Verification items for the finished model (mm, model axes). Face numbers are marked on the shaded views. Round coordinates to 2 decimals unless told otherwise and drop trailing zeros. Order: outer loops, then holes, each group sorted by start corner. A loop starts at its lowest first (then second) coordinate and runs counter-clockwise, first axis right, second up.
Autodesk Inventor part; units mm, degrees
ref_plane "Work Plane6" through (1000, 0, 0) normal (1, 0, 0) x (0, 0, -1)
ref_plane "Work Plane7" through (0, 775, 0) normal (0, 1, 0) x (1, 0, 0)
ref_plane "Work Plane8" through (0, 237, 0) normal (0, -1, 0) x (1, 0, 0)
sketch "Sketch1" plane through (0, 0, 0) normal (0, 0, 1) x (1, 0, 0)
  line L0 (0, 0) -> (1000, 0)
  line L1 (1000, 0) -> (1000, 1000)
  line L2 (1000, 1000) -> (0, 1000)
  line L3 (0, 1000) -> (0, 0)
  dimension "d0" = 1000
  dimension "d1" = 1000
extrude "Extrusion1" add sketch "Sketch1" along normal blind 100
sketch "Sketch8" plane through (0, 0, 100) normal (0, 0, 1) x (1, 0, 0)
  line L0 (1000, 1000) -> (0, 1000)
  line L1 (0, 1000) -> (150, 1000)
  line L2 (150, 1000) -> (150, 850)
  circle A0 centre (150, 850) radius 12.5
  point P0 (0, 0)
  dimension "d30" = 150
  dimension "d31" = 150
  dimension "d32" = 25
extrude "Extrusion4" cut sketch "Sketch8" against normal blind 100
sketch "Sketch9" plane through (0, 0, 100) normal (0, 0, 1) x (1, 0, 0)
  line L0 (425, 260) -> (765, 260)
  line L1 (765, 260) -> (765, 50)
  line L2 (765, 50) -> (425, 50)
  line L3 (425, 50) -> (425, 260)
  line L4 (0, 0) -> (1000, 0)
  line L5 (0, 1000) -> (0, 0)
  dimension "d35" = 210
  dimension "d36" = 340
  dimension "d37" = 50
extrude "Extrusion5" add sketch "Sketch9" along normal blind 115
ref_plane "Work Plane6" through (1000, 0, 0) normal (1, 0, 0) x (0, 0, -1)
ref_plane "Work Plane7" through (0, 775, 0) normal (0, 1, 0) x (1, 0, 0)
sketch "Sketch12" plane through (0, 0, 100) normal (0, 0, 1) x (1, 0, 0)
  line L0 (0, 0) -> (1000, 0)
  line L1 (877, 141) -> (742, 141) construction
  line L2 (877, 141) -> (877, 166) construction
  line L3 (902, 166) -> (902, 116)
  line L4 (902, 116) -> (852, 116)
  line L5 (852, 116) -> (852, 166)
  line L6 (852, 166) -> (902, 166)
  dimension "d58" = 25
  dimension "d59" = 50
  dimension "d60" = 50
  dimension "d63" = 25
  dimension "d64" = 25
extrude "Extrusion8" add sketch "Sketch12" along normal blind 0.5
ref_plane "Work Plane8" through (0, 237, 0) normal (0, -1, 0) x (1, 0, 0)
sketch "Sketch13" plane through (0, 0, 100) normal (0, 0, 1) x (1, 0, 0)
  line L0 (425, 260) -> (425, 50)
  line L1 (425, 155) -> (395, 155)
  line L2 (395, 155) -> (395, 160)
  line L3 (395, 160) -> (220, 160)
  line L4 (220, 160) -> (220, 130)
  line L5 (220, 130) -> (395, 130)
  line L6 (395, 130) -> (395, 155)
  line L7 (425, 50) -> (164, 50)
  point P0 (0, 0)
  dimension "d67" = 30
  dimension "d68" = 5
  dimension "d69" = 175
  dimension "d73" = 80
extrude "Extrusion9" cut sketch "Sketch13" against normal blind 1
sketch "Sketch14" plane through (0, 0, 100) normal (0, 0, 1) x (1, 0, 0)
  line L0 (580, 520) -> (380, 520)
  line L1 (380, 520) -> (380, 700)
  line L2 (380, 700) -> (580, 700)
  line L3 (580, 700) -> (580, 520)
  line L4 (0, 1000) -> (0, 0)
  line L5 (1000, 1000) -> (0, 1000)
  point P0 (380, 610)
  dimension "d74" = 180
  dimension "d75" = 200
  dimension "d76" = 380
  dimension "d77" = 300
extrude "Extrusion10" cut sketch "Sketch14" against normal blind 1
sketch "Sketch16" plane through (0, 0, 100) normal (0, 0, 1) x (1, 0, 0)
  line L0 (722.7051, 770) -> (822.7051, 770)
  line L1 (822.7051, 770) -> (822.7051, 800)
  line L2 (822.7051, 800) -> (722.7051, 800)
  line L3 (722.7051, 800) -> (722.7051, 770)
  line L4 (1000, 1000) -> (0, 1000)
  point P0 (0, 0)
  dimension "d86" = 100
  dimension "d87" = 30
  dimension "d90" = 200
extrude "Extrusion12" cut sketch "Sketch16" against normal blind 3
sketch "Sketch18" plane through (0, 0, 100) normal (0, 0, 1) x (1, 0, 0)
  line L0 (950, 500) -> (750, 500)
  line L1 (750, 500) -> (750, 520)
  line L2 (750, 520) -> (950, 520)
  line L3 (950, 520) -> (950, 500)
  line L4 (1000, 0) -> (1000, 1000)
  line L5 (0, 0) -> (1000, 0)
  dimension "d93" = 20
  dimension "d94" = 50
  dimension "d95" = 500
  dimension "d96" = 200
extrude "Extrusion14" add sketch "Sketch18" along normal blind 1
properties part number "Base"
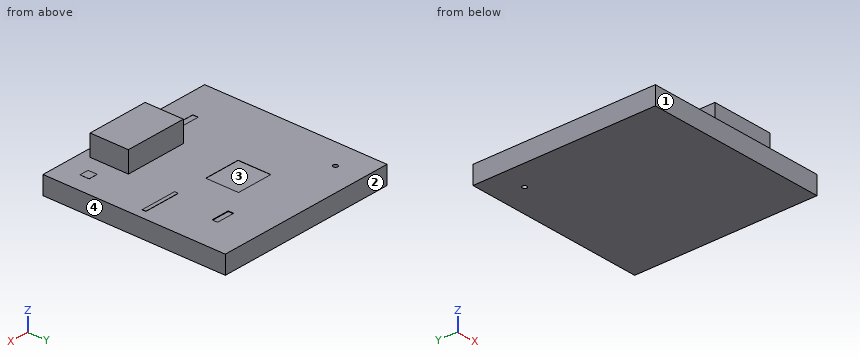
1) Draft check along Y on the marked faces 1, 2, 3 and 4. Enter one of: released by +Y, released by -Y, zero draft, split by the parting line, or undercut.
2) Scan lines: probe 1 along X at (y, z) = (850, 37.5); probe 2 along Y at (x, z) = (150, 64); probe 3 along Z at (x, y) = (373.5, 600). Record each from-to range of solid material in increasing order.
3) Sectioned sample at C-C on x = 302. Record the cut outline in (y, z), then the cut area to 4 significant figures.
4) Sectioned sample at A-A on y = 850. Record the cut outline in (x, z).
5) Go/stop test with flat-tipped pins: pin 1 Ø8 at (x, z) = (518, 173.5) entering from -Y; pin 2 Ø10 at (x, y) = (879.5, 250.5) entering from -Z; pin 3 Ø1 at (x, y) = (501, 677) entering from +Z. Record where each tip stops, or that it passes through.
6) Sectioned sample at D-D on z = 174. Record the cut outline in (x, y).
7) Sectioned sample at B-B on x = 150. Record the cut outline in (y, z), then the cut area to 3 significant figures.
Returned:
1. face 1: released by -Y
1. face 2: released by +Y
1. face 3: undercut
1. face 4: zero draft
2. probe 1: x = 0 to 137.5, 162.5 to 1000
2. probe 2: y = 0 to 837.5, 862.5 to 1000
2. probe 3: z = 0 to 100
3. outline: (0, 0) - (1000, 0) - (1000, 100) - (160, 100) - (160, 99) - (130, 99) - (130, 100) - (0, 100) - close
3. area: 100,000 mm2
4. outline: (0, 0) - (137.5, 0) - (137.5, 100) - (0, 100) - close; (162.5, 0) - (1000, 0) - (1000, 100) - (162.5, 100) - close
5. pin 1: stops at y = 50
5. pin 2: stops at z = 0
5. pin 3: stops at z = 99
6. outline: (425, 50) - (765, 50) - (765, 260) - (425, 260) - close
7. outline: (0, 0) - (837.5, 0) - (837.5, 100) - (0, 100) - close; (862.5, 0) - (1000, 0) - (1000, 100) - (862.5, 100) - close
7. area: 97,500 mm2
